```python
from build123d import *

# Parameters (mm, degrees)
F0_W     = 23.4994404018
F0_H     = 65.5540376902
F1_DEPTH = 25.4
F3_DEPTH = 61.722
F4_R     = 11.3020166748
F5_DEPTH = 63.754


with BuildPart() as f1:
    # F0 (on Right) → F1 (new body)
    with BuildSketch(Plane.YZ):
        Polygon((0, 65.5540376902), (0, 0), (51.2884631753, 0), align=None)
        with Locations((-11.7497202009, 32.7770188451)):
            Rectangle(F0_W, F0_H)
    extrude(amount=F1_DEPTH)

    # F2 (on face) → F3 (join)
    with BuildSketch(Plane.YZ.offset(25.4)):
        Polygon((0, 58.6534105241), (-23.4994404018, 58.6534105241), (-23.4994404018, 0), (44.9473448098, 0), align=None)
    extrude(amount=F3_DEPTH)

    # F4 (on face) → F5 (cut)
    with BuildSketch(Plane(origin=(0, 28.3177833218, 21.7005142555), x_dir=(-1, 0, 0), z_dir=(0, 0.7937387929, 0.6082587678))):
        with Locations((-58.4767535329, 14.2394453287)):
            Circle(F4_R)
    extrude(amount=-F5_DEPTH, mode=Mode.SUBTRACT)


solid = f1.part
```
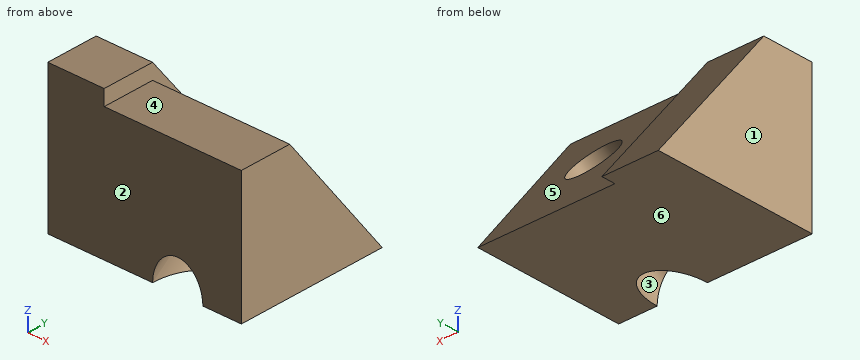
Geometry check sheet. Reference: the model listing, model coordinates, mm. Face numbers are marked on the shaded views. A direction names the side the tool comes from. Coordinates: 2 decimals unless noted, no trailing zeros. Order: outer loops, then holes, each group sorted by start corner. A loop starts at its lowest first (then second) coordinate and runs counter-clockwise, first axis right, second up.
Q1. Draft check along X on the marked faces 1, 2 and 3. Enter one of: released by +X, released by -X, zero draft, split by the parting line, or undercut.
Reply:
face 1: released by -X
face 2: zero draft
face 3: undercut
Q2. Depth check by flat-ended pin: pin 1 Ø8 at (x, y) = (30, 43.5) entering from -Z; pin 2 Ø1.5 at (x, y) = (66.5, 40) entering from +Z; pin 3 Ø8 at (x, z) = (73, 49.5) entering from +Y; pin 4 Ø10 at (x, z) = (26.5, 32.5) entering from +Y. Enter the tip coordinate at first touch or a pass-through.
Reply:
pin 1: stops at z = 0
pin 2: stops at z = 7.43
pin 3: stops at y = 10.08
pin 4: stops at y = 29.68
Q3. Thickness scan on probe 1 along X at (y, z) = (-12.5, 10.5); probe 2 along Z at (x, y) = (68, 12); probe 3 along X at (y, z) = (13.5, 23). Record the ranges inside material, lowest first.
Reply:
probe 1: x = 0 to 47.3, 69.65 to 87.12
probe 2: z = 0 to 19.47, 34.8 to 42.99
probe 3: x = 0 to 47.98, 68.97 to 87.12
Q4. Sectioned sample at A-A on x = 61.5. Record the cut outline in (y, z).
Reply:
outline: (-23.5, 13.65) - (13.03, 41.65) - (0, 58.65) - (-23.5, 58.65) - close; (-5.51, 0) - (44.95, 0) - (26.28, 24.36) - close
Q5. Tool access check on the marked faces 4, 5 and 6. Record the directions out of +Z, -Z, +X, -X, +Y, -Y that give a thin tool (end or side, any length) a straight path to the whole face; none if there is none.
Reply:
face 4: +Z, +X, +Y, -Y
face 5: +Z, +X, +Y
face 6: -Z, +X, -X, +Y, -Y
Q6. Sectioned sample at B-B on y = 41.5. Record the cut outline in (x, z), and give its area (3 significant figures).
Reply:
outline: (0, 0) - (87.12, 0) - (87.12, 4.5) - (25.4, 4.5) - (25.4, 12.51) - (0, 12.51) - close
area: 595 mm2
Q7. Sectioned sample at C-C on x = 75.5. Record the cut outline in (y, z), and give its area (3 significant figures).
Reply:
outline: (-23.5, 0) - (44.95, 0) - (0, 58.65) - (-23.5, 58.65) - close
area: 2,700 mm2
Q8. Sectioned sample at D-D on z = 47.5. Record the cut outline in (x, y).
Reply:
outline: (0, -23.5) - (87.12, -23.5) - (87.12, 8.55) - (25.4, 8.55) - (25.4, 14.13) - (0, 14.13) - close
